Could you check a few things on this drawing? It's one solid part, dimensions in mm from its lowest x, y, z. A direction names the side the tool comes from. Round coordinates to 2 decimals unless told otherwise and drop trailing zeros. Write each loop counter-clockwise with the first axis right and the second up, starting at its lowest first coordinate (ties: lowest second). Pieces come first, ordered by that corner, then holes. Notation, with made-up numbers: (-9, 35) - (33, 35) arc R28 ccw to (33, 54) - close; hole circle Ø1 at (10, 19.25). An arc over 180 degrees is marked (long way). Put each result on its own line as item: value.
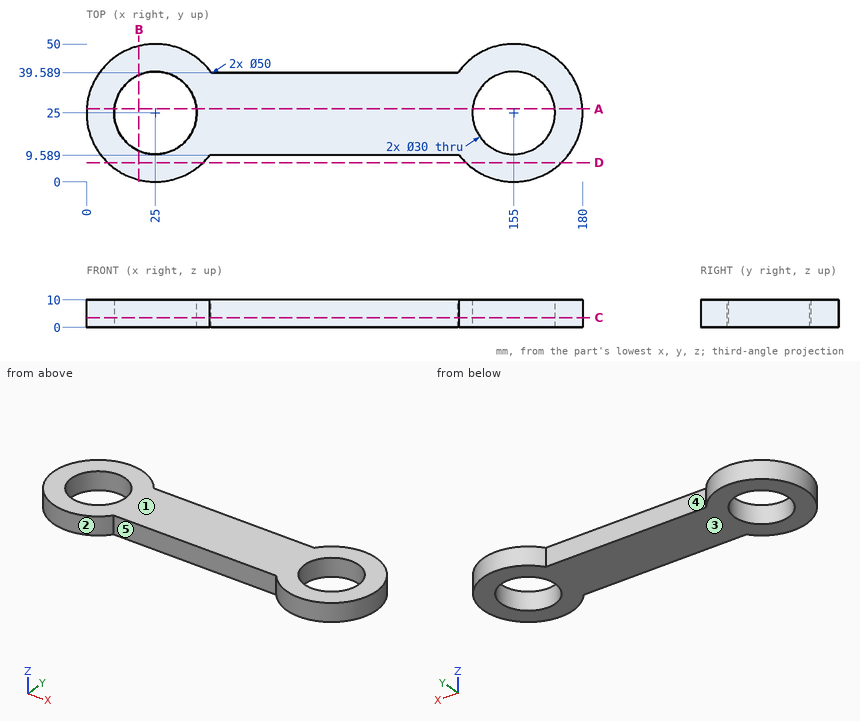
(1) Imagine slicing it at B-B, the plane x = 19. List the corners of the cut face in (y, z) for me.
Values found:
outline: (0.73, 0) - (11.25, 0) - (11.25, 10) - (0.73, 10) - close; (38.75, 0) - (49.27, 0) - (49.27, 10) - (38.75, 10) - close
(2) Imagine slicing it at C-C, the plane z = 3.5. List the corners of the cut face in (x, y) for me (1 decimal), then the cut area to 3 significant figures.
Values found:
outline: (44.7, 9.6) - (135.3, 9.6) arc R25 ccw (long way) to (134.7, 39.6) - (45.3, 39.6) arc R25 ccw (long way) to start; hole circle Ø30 at (25, 25); hole circle Ø30 at (155, 25)
area: 5,010 mm^2
(3) For the marked faces 3, 4 and 5, which set-ups out of +Z, -Z, +X, -X, +Y, -Y let a thin tool reach every point of the face, with its end or its side?
Values found:
face 3: -Z, +X, -X, +Y, -Y
face 4: +Z, -Z, +Y
face 5: +Z, -Z, -Y
(4) Please list where these lines run through material, in increasing order: probe 1 along X at (y, z) = (25.5, 4.5) (1 decimal); probe 2 along X at (y, z) = (29, 4.5); probe 3 along X at (y, z) = (9.5, 0.75) (1 decimal). Write a range as from..to.
Values found:
probe 1: x = 0..10, 40..140, 170..180
probe 2: x = 0.32..10.54, 39.46..140.54, 169.46..179.68
probe 3: x = 5.4..44.6, 135.4..174.6
(5) Imagine slicing it at A-A, the plane y = 26.5. List the corners of the cut face in (x, z) for me (1 decimal), then the cut area to 3 significant figures.
Values found:
outline: (0, 0) - (10.1, 0) - (10.1, 10) - (0, 10) - close; (39.9, 0) - (140.1, 0) - (140.1, 10) - (39.9, 10) - close; (169.9, 0) - (180, 0) - (180, 10) - (169.9, 10) - close
area: 1,200 mm^2
(6) I'm going to push flat-ended pins straight in: pin 1 (2 mm diameter, centred on y = 38.5, z = 5, fed in from -X); pin 2 (3 mm diameter, centred on x = 77, z = 3.5, fed in from +Y); pin 3 (5 mm diameter, centred on y = 8.5, z = 3.5, fed in from -X). Where does each tip first touch, or does it pass through?
Values found:
pin 1: stops at x = 3.35
pin 2: stops at y = 39.59
pin 3: stops at x = 4.29
(7) If we mould it in two halves opening along X, with no side actions, what happens to the marked faces 1 and 2? For each: pulls with the +X half, pulls with the -X half, needs draft (parallel to the pull), parting line crosses it, or undercut.
Values found:
face 1: needs draft
face 2: undercut
(8) Imagine slicing it at D-D, the plane y = 7. List the corners of the cut face in (x, z) for me.
Values found:
outline: (7.65, 0) - (42.35, 0) - (42.35, 10) - (7.65, 10) - close; (137.65, 0) - (172.35, 0) - (172.35, 10) - (137.65, 10) - close
